Design review of the part built by this model. Coordinates are the model's own, in mm. Coordinates: 2 decimals unless noted, no trailing zeros. Order: outer loops, then holes, each group sorted by start corner. A loop starts at its lowest first (then second) coordinate and runs counter-clockwise, first axis right, second up. Notation, with made-up numbers: M 11,-31 L 36,-31 A26 cw 36,3 Z; hole C 81.25,20 d7. An arc over 180 degrees is marked long. Use CSV: the item, a comma, the result in double quotes.
```python
from build123d import *

# Parameters (mm, degrees)
SKETCH1_W           = 40
SKETCH1_H           = 20
SKETCH1_W_2         = 36
SKETCH1_H_2         = 16
BOSS_EXTRUDE1_DEPTH = 400
SKETCH2_R           = 4
CUT_EXTRUDE1_DEPTH  = 403.49223595
BOSS_EXTRUDE2_DEPTH = 2
SKETCH4_R           = 4
CUT_EXTRUDE2_DEPTH  = 409.931534612
SKETCH5_R           = 4
CUT_EXTRUDE3_DEPTH  = 409.931534612
CUT_EXTRUDE4_START  = -2
SKETCH7_W           = 36
SKETCH7_H           = 150
CUT_EXTRUDE4_DEPTH  = 2
SKETCH8_W           = 40
SKETCH8_H           = 20
SKETCH8_W_2         = 36
SKETCH8_H_2         = 16
BOSS_EXTRUDE3_DEPTH = 200


with BuildPart() as part:
    # Sketch1 → Boss-Extrude1 (new body)
    with BuildSketch(Plane.XY):
        with Locations((20, -10)):
            Rectangle(SKETCH1_W, SKETCH1_H)
        with Locations((20, -10)):
            Rectangle(SKETCH1_W_2, SKETCH1_H_2, mode=Mode.SUBTRACT)
    extrude(amount=BOSS_EXTRUDE1_DEPTH)

    # Sketch2 → Cut-Extrude1 (cut, through all)
    with BuildSketch(Plane(origin=(40, 0, 0), x_dir=(0, 0, -1), z_dir=(1, 0, 0))):
        with Locations((-10, -9)):
            Circle(SKETCH2_R)
        with Locations((-40, -9)):
            Circle(SKETCH2_R)
        with Locations((-70, -9)):
            Circle(SKETCH2_R)
    extrude(amount=-CUT_EXTRUDE1_DEPTH, mode=Mode.SUBTRACT)

    # Sketch3 → Boss-Extrude2 (add)
    with BuildSketch(Plane(origin=(40, 0, 0), x_dir=(0, 0, -1), z_dir=(1, 0, 0))):
        with BuildLine():
            Line((-400, 0), (-250, 0))
            ThreePointArc((-250, 0), (-325, 75), (-400, 0))
        make_face()
    boss_extrude2 = extrude(amount=-BOSS_EXTRUDE2_DEPTH)

    # Mirror1: Boss-Extrude2 across plane
    add(boss_extrude2.mirror(Plane(origin=(20, 0, 0), x_dir=(0, 0, 1), z_dir=(1, 0, 0))))

    # Sketch4 → Cut-Extrude2 (cut, through all)
    with BuildSketch(Plane(origin=(40, 0, 0), x_dir=(0, 0, -1), z_dir=(1, 0, 0))):
        with Locations((-390, 0)):
            Circle(SKETCH4_R)
        with Locations((-388.751043226, 12.680870931)):
            Circle(SKETCH4_R)
        with Locations((-385.052169613, 24.874423104)):
            Circle(SKETCH4_R)
        with Locations((-379.0455248, 36.112065146)):
            Circle(SKETCH4_R)
        with Locations((-370.961940777, 45.961940777)):
            Circle(SKETCH4_R)
        with Locations((-361.112065146, 54.0455248)):
            Circle(SKETCH4_R)
        with Locations((-349.874423104, 60.052169613)):
            Circle(SKETCH4_R)
        with Locations((-337.680870931, 63.751043226)):
            Circle(SKETCH4_R)
        with Locations((-325, 65)):
            Circle(SKETCH4_R)
        with Locations((-312.319129069, 63.751043226)):
            Circle(SKETCH4_R)
        with Locations((-300.125576896, 60.052169613)):
            Circle(SKETCH4_R)
        with Locations((-288.887934854, 54.0455248)):
            Circle(SKETCH4_R)
        with Locations((-279.038059223, 45.961940777)):
            Circle(SKETCH4_R)
        with Locations((-270.9544752, 36.112065146)):
            Circle(SKETCH4_R)
        with Locations((-264.947830387, 24.874423104)):
            Circle(SKETCH4_R)
        with Locations((-261.248956774, 12.680870931)):
            Circle(SKETCH4_R)
        with Locations((-260, 0)):
            Circle(SKETCH4_R)
    extrude(amount=-CUT_EXTRUDE2_DEPTH, mode=Mode.SUBTRACT)

    # Sketch5 → Cut-Extrude3 (cut, through all)
    with BuildSketch(Plane(origin=(40, 0, 0), x_dir=(0, 0, -1), z_dir=(1, 0, 0))):
        with Locations((-325, 0)):
            Circle(SKETCH5_R)
    extrude(amount=-CUT_EXTRUDE3_DEPTH, mode=Mode.SUBTRACT)

    # Sketch7 → Cut-Extrude4 (cut)
    with BuildSketch(Plane(origin=(0, 0, 0), x_dir=(1, 0, 0), z_dir=(0, 1, 0)).offset(CUT_EXTRUDE4_START)):
        with Locations((20, -325)):
            Rectangle(SKETCH7_W, SKETCH7_H)
    extrude(amount=CUT_EXTRUDE4_DEPTH, mode=Mode.SUBTRACT)

    # Sketch8 → Boss-Extrude3 (add)
    with BuildSketch(Plane(origin=(0, 0, 0), x_dir=(-1, 0, 0), z_dir=(0, 0, -1))):
        with Locations((-20, -10)):
            Rectangle(SKETCH8_W, SKETCH8_H)
        with Locations((-20, -10)):
            Rectangle(SKETCH8_W_2, SKETCH8_H_2, mode=Mode.SUBTRACT)
    extrude(amount=BOSS_EXTRUDE3_DEPTH)


solid = part.part
```
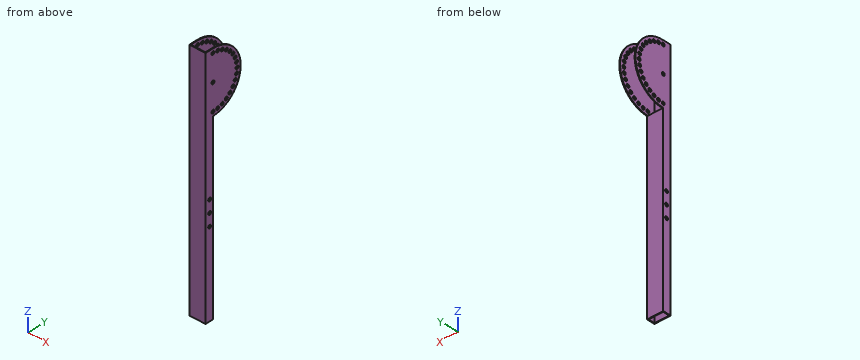
(1) Add section A-A on x = 7. State the section outline as (y, z) points.
The answers:
outline,"M -20,-200 L -18,-200 L -18,400 L -20,400 Z; M -2,-200 L 0,-200 L 0,250 L -2,250 Z"
(2) Wall thickness on probe 1 along Y at (x, z) = (35, -102.5); probe 2 along X at (y, z) = (61, 281.5); probe 3 along Y at (x, z) = (26, 289.5): over which ranges is each line inside the solid? List them lowest first.
The answers:
probe 1,"y = -20 to -18, -2 to 0"
probe 2,"x = 0 to 2, 38 to 40"
probe 3,"y = -20 to -18"
(3) Add section B-B on z = 176. State the section outline as (x, y) points, and give its area (3 significant figures).
The answers:
outline,"M 0,-20 L 40,-20 L 40,0 L 0,0 Z; hole M 2,-18 L 38,-18 L 38,-2 L 2,-2 Z"
area,"224 mm2"
(4) Clearance check with flat-ended pins moving along their axes: P1, Ø8, axis at x = 11.5, z = 176, coming from the +Y side; P2, Ø2, axis at x = 28, y = -1.5, coming from the +Z side. State where each tip first meets the part, or that it passes through.
The answers:
P1,"stops at y = 0"
P2,"stops at z = 250"
